from build123d import *

# Parameters (mm, degrees)
SKETCH4_R               = 3.175
BOSS_EXTRUDE2_DEPTH     = 25.4
FILLET1_R               = 5.08
M5_CLEARANCE_HOLE1_D    = 5.6
CUT_EXTRUDE1_DEPTH      = 32.908355123
CUT_EXTRUDE1_DEPTH_BACK = 32.908355123
SKETCH9_W               = 6.985
SKETCH9_H               = 10.16
SKETCH10_R              = 1.27
CUT_EXTRUDE2_DEPTH      = 55.347245805
CHAMFER1_SIZE           = 0.7112


with BuildPart() as part:
    # Sketch4 → Boss-Extrude2 (new, symmetric)
    with BuildSketch(Plane.XY):
        Circle(SKETCH4_R)
        with BuildLine():
            Line((19.050000043, -1.905), (19.050000043, -0.4826))
            Line((19.050000043, -0.4826), (3.138108067, -0.4826))
            ThreePointArc((3.138108067, -0.4826), (2.926778646, -1.230687513), (2.54, -1.905))
            Line((2.54, -1.905), (19.050000043, -1.905))
        make_face()
    extrude(amount=BOSS_EXTRUDE2_DEPTH, both=True)

    # Fillet1
    fillet1_edges = [part.edges().sort_by_distance(p)[0] for p in [
        (2.54, -1.905, 0),
    ]]
    fillet(fillet1_edges, radius=FILLET1_R)

    # M5 Clearance Hole1 (through all)
    with Locations(Plane(origin=(0, -0.4826, 0), x_dir=(1, 0, 0), z_dir=(0, 1, 0))):
        with Locations((11.938000043, 18.288), (11.938000043, -18.288)):
            Hole(M5_CLEARANCE_HOLE1_D / 2)

    # Sketch9 → Cut-Extrude1 (cut, two sides: drawn at the far end of the back side and taken through both)
    with BuildSketch(Plane(origin=(0, 0, 0), x_dir=(1, 0, 0), z_dir=(0, 1, 0)).offset(-CUT_EXTRUDE1_DEPTH_BACK)):
        with Locations((0.3175, 10.16)):
            Rectangle(SKETCH9_W, SKETCH9_H)
        with Locations((0.3175, -10.16)):
            Rectangle(SKETCH9_W, SKETCH9_H)
    extrude(amount=CUT_EXTRUDE1_DEPTH + CUT_EXTRUDE1_DEPTH_BACK, mode=Mode.SUBTRACT)

    # Sketch10 → Cut-Extrude2 (cut, through all)
    with BuildSketch(Plane.XY.offset(25.4)):
        Circle(SKETCH10_R)
    extrude(amount=-CUT_EXTRUDE2_DEPTH, mode=Mode.SUBTRACT)

    # Chamfer1
    chamfer1_edges = [part.edges().sort_by_distance(p)[0] for p in [
        (14.738000043, -0.4826, 18.288),
        (14.738000043, -0.4826, -18.288),
    ]]
    chamfer(chamfer1_edges, length=CHAMFER1_SIZE)


solid = part.part
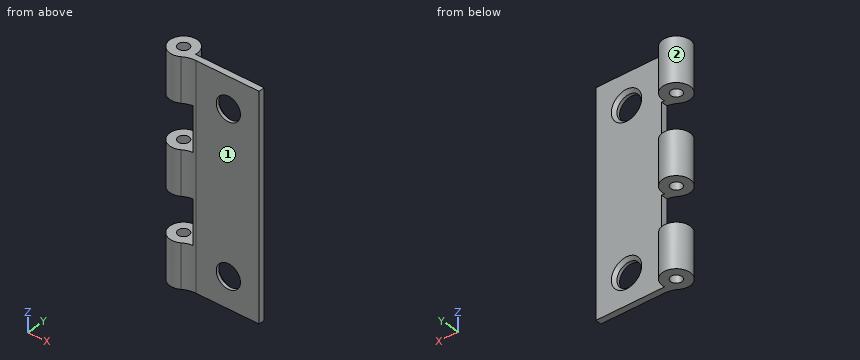
Part model, mm, in its own coordinate system. Face numbers are marked on the shaded views. A direction names the side the tool comes from. Coordinates: 2 decimals unless noted, no trailing zeros. Write each loop counter-clockwise with the first axis right and the second up, starting at its lowest first coordinate (ties: lowest second). Pieces come first, ordered by that corner, then holes. Notation, with made-up numbers: M 14,13 L 23,13 A29 ccw 23,39 Z; hole C -37,-23 d7. An arc over 180 degrees is marked long. Return JSON: item names as keys, results as strings.
1. Saw through at B-B, the plane z = -3. Write the cut outline in (x, y) (3 decimals), then the cut area to 3 significant figures.
Determined:
{"outline": "M 1.692,-2.687 A5.08 cw 4.399,-1.905 L 19.05,-1.905 L 19.05,-0.483 L 3.138,-0.483 A3.175 ccw long Z; hole C 0,0 d2.54", "area": "49.9 mm²"}
2. Saw through at C-C, the plane y = 0.5. Write the cut outline in (x, z), then the cut area to 3 significant figures.
Determined:
{"outline": "M -3.14,-25.4 L -1.17,-25.4 L -1.17,-15.24 L -3.14,-15.24 Z; M -3.14,-5.08 L -1.17,-5.08 L -1.17,5.08 L -3.14,5.08 Z; M -3.14,15.24 L -1.17,15.24 L -1.17,25.4 L -3.14,25.4 Z; M 1.17,-25.4 L 3.14,-25.4 L 3.14,-15.24 L 1.17,-15.24 Z; M 1.17,-5.08 L 3.14,-5.08 L 3.14,5.08 L 1.17,5.08 Z; M 1.17,15.24 L 3.14,15.24 L 3.14,25.4 L 1.17,25.4 Z", "area": "120 mm²"}
3. 3-axis set-ups, long thin cutter, end or side, ignore diameter. For the marked faces 1 and 2: which of +Z, -Z, +X, -X, +Y, -Y reach the whole face in a straight line?
Determined:
{"face 1": "+Z, -Z, +X, -Y", "face 2": "+Z, -Z"}
4. Probe L1, parallel to Z at x = -1.75, y = 2.25; L2, parallel to Z at x = 14, y = -1.5; L3, parallel to Y at x = 0, z = -20.5 (3 decimals). List the from-to ranges inside material, lowest first.
Determined:
{"L1": "-25.4 to -15.24, -5.08 to 5.08, 15.24 to 25.4", "L2": "-25.4 to -20.18, -16.39 to 16.39, 20.18 to 25.4", "L3": "-3.175 to -1.27, 1.27 to 3.175"}
5. Flat gauge pins, fed straight in: pin 1 Ø4 at (x, z) = (15, 12.5) entering from +Y; pin 2 Ø10 at (x, z) = (11.5, -17) entering from -Y (3 decimals); pin 3 Ø11.5 at (x, z) = (8, -3.5) entering from -Y. Where does each tip first touch, or does it go through?
Determined:
{"pin 1": "y = -0.48", "pin 2": "y = -1.905", "pin 3": "y = -2.38"}
6. Saw through at D-D, the plane z = -9. Write the cut outline in (x, y) (3 decimals), then the cut area to 3 significant figures.
Determined:
{"outline": "M 3.81,-1.939 A5.08 cw 4.399,-1.905 L 19.05,-1.905 L 19.05,-0.483 L 3.81,-0.483 Z", "area": "21.7 mm²"}
7. Saw through at A-A, the plane x = 0. Write the cut outline in (y, z) (3 decimals), then the cut area to 3 significant figures.
Determined:
{"outline": "M -3.175,-25.4 L -1.27,-25.4 L -1.27,-15.24 L -3.175,-15.24 Z; M -3.175,-5.08 L -1.27,-5.08 L -1.27,5.08 L -3.175,5.08 Z; M -3.175,15.24 L -1.27,15.24 L -1.27,25.4 L -3.175,25.4 Z; M 1.27,-25.4 L 3.175,-25.4 L 3.175,-15.24 L 1.27,-15.24 Z; M 1.27,-5.08 L 3.175,-5.08 L 3.175,5.08 L 1.27,5.08 Z; M 1.27,15.24 L 3.175,15.24 L 3.175,25.4 L 1.27,25.4 Z", "area": "116 mm²"}
